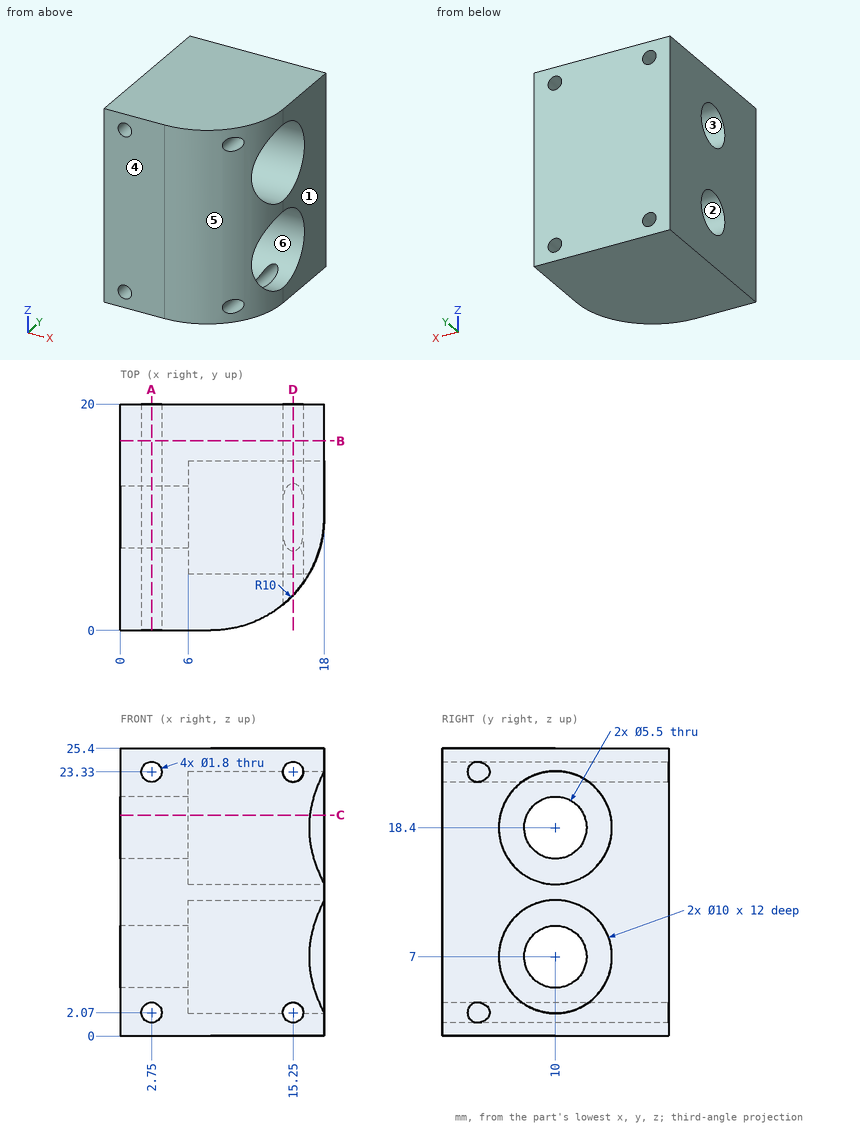
Here's the drawing with two shaded views (mm, measured from the low corner). I have some questions. A direction names the side the tool comes from. Give positions to 0.01 mm unless a question says otherwise; leave off trailing zeros. Order: outer loops, then holes, each group sorted by start corner. A loop starts at its lowest first (then second) coordinate and runs counter-clockwise, first axis right, second up. Notation, with made-up numbers: M 36,-30.75 L 47,-30.75 A13 cw 47,-6.75 Z; hole C 5.5,32 d8. An arc over 180 degrees is marked long. One line per item, written item: value.
1) We'd pull the mould along Y, two halves only. Please class the marked faces 1, 2, 3 and 4: released by +Y, released by -Y, zero draft, split by the parting line, or undercut.
Answer sheet:
face 1: zero draft
face 2: undercut
face 3: undercut
face 4: released by -Y
2) On a 3-axis mill with a long thin cutter (end or side, diameter ignored), from which of +Z, -Z, +X, -X, +Y, -Y can I reach the whole of each face in a straight line? I mean the marked faces 5 and 6. Say none if no direction works.
Answer sheet:
face 5: +Z, -Z, +X, -Y
face 6: +X
3) For P1, Ø3, axis at x = 15.25, z = 23.33, coming from the -Y side; P2, Ø9, axis at y = 10, z = 18.4, coming from the +X side, each with a flat end and sliding along its axis, tell me the tip position at first contact or that it passes through.
Answer sheet:
P1: stops at y = 1.82
P2: stops at x = 6
4) I want a section at D-D, the plane x = 15.25. List the corners of the cut face in (y, z) for me, plus the area to 3 significant figures.
Answer sheet:
outline: M 3.11,0 L 20,0 L 20,1.17 L 3.11,1.17 Z; M 3.11,2.97 L 7.04,2.97 A5 cw long 12.96,2.97 L 20,2.97 L 20,22.43 L 12.96,22.43 A5 cw long 7.04,22.43 L 3.11,22.43 Z; M 3.11,24.23 L 20,24.23 L 20,25.4 L 3.11,25.4 Z
area: 219 mm^2
5) I want a section at A-A, the plane x = 2.75. List the corners of the cut face in (y, z) for me.
Answer sheet:
outline: M 0,0 L 20,0 L 20,1.17 L 0,1.17 Z; M 0,2.97 L 20,2.97 L 20,22.43 L 0,22.43 Z; M 0,24.23 L 20,24.23 L 20,25.4 L 0,25.4 Z; hole C 10,7 d5.5; hole C 10,18.4 d5.5
6) Please list where these lines run through material, in increasing order: line 1 along X through (y, z) = (13.25, 1.75); line 2 along Y through (x, z) = (3.6, 18.4); line 3 along Z through (x, y) = (1.75, 8.25).
Answer sheet:
line 1: x = 0 to 1.91, 3.59 to 14.41, 16.09 to 18
line 2: y = 0 to 7.25, 12.75 to 20
line 3: z = 0 to 4.88, 9.12 to 16.28, 20.52 to 25.4
7) I want a section at B-B, the plane y = 16.75. List the corners of the cut face in (x, z) for me, plus the area to 3 significant figures.
Answer sheet:
outline: M 0,0 L 18,0 L 18,25.4 L 0,25.4 Z; hole C 2.75,2.07 d1.8; hole C 2.75,23.33 d1.8; hole C 15.25,2.07 d1.8; hole C 15.25,23.33 d1.8
area: 447 mm^2
8) I want a section at C-C, the plane z = 19.5. List the corners of the cut face in (x, y) for me, plus the area to 3 significant figures.
Answer sheet:
outline: M 0,0 L 8,0 A10 ccw 16.73,5.12 L 6,5.12 L 6,7.48 L 0,7.48 Z; M 0,12.52 L 6,12.52 L 6,14.88 L 18,14.88 L 18,20 L 0,20 Z
area: 193 mm^2
